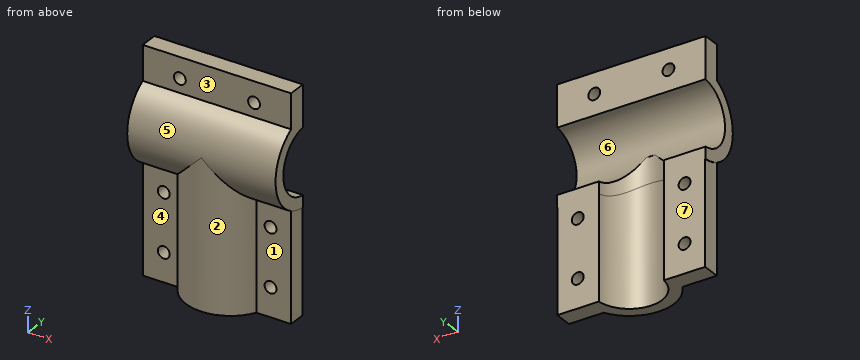
Autodesk Inventor part; units mm, degrees
ref_plane "YZ Plane" through (0, 0, 0) normal (1, 0, 0) x (0, 1, 0)
ref_plane "XZ Plane" through (0, 0, 0) normal (0, 1, 0) x (-1, 0, 0)
ref_plane "XY Plane" through (0, 0, 0) normal (0, 0, 1) x (1, 0, 0)
sketch "Sketch1" plane through (0, 0, 0) normal (1, 0, 0) x (0, 1, 0)
  arc A0 (-1, 14.96663) -> (0, -15) centre (0, 0) ccw
  arc A1 (-1, 10.954451) -> (0, -11) centre (0, 0) ccw
  line L0 (0, 15) -> (0, -15)
  line L1 (-1, 14.96663) -> (-1, 10.954451)
  point P0 (0, 11.5)
  dimension "d0" = 30
  dimension "d1" = 22
extrude "Extrusion1" add sketch "Sketch1" along normal blind 50
sketch "Sketch2" plane through (50, 0, 0) normal (1, 0, 0) x (0, 0, -1)
  line L0 (-10.954451, -1) -> (-14.96663, -1)
  line L1 (-14.96663, -1) -> (-24.96663, -1)
  line L2 (-24.96663, -1) -> (-24.96663, -7)
  line L3 (-24.96663, -7) -> (-13.211534, -7)
  arc A0 (-14.96663, -1) -> (15, 0) centre (0, 0) ccw
  line L4 (-14.96663, -1) -> (-13.211534, -7)
  point P0 (-13.266499, -7)
  dimension "d5" = 10
  dimension "d6" = 6
extrude "Extrusion2" add sketch "Sketch2" against normal blind 50 contours A0 L3 L2 L1
sketch "Sketch3" plane through (0, 0, 0) normal (0, 1, 0) x (-1, 0, 0)
  line L0 (0, 0) -> (-25, 0) construction
  line L1 (-25, 0) -> (-25, -50) construction
  dimension "d9" = 25
  dimension "d10" = 50
ref_plane "Work Plane1" through (25, 0, -50) normal (0, 0, -1) x (-1, 0, 0)
sketch "Sketch4" plane through (25, 0, -50) normal (0, 0, -1) x (-1, 0, 0)
  line L0 (25, 0) -> (-25, 0)
  arc A0 (-10.954451, -1) -> (10.954451, -1) centre (0, 0) ccw
  arc A1 (-14.96663, -1) -> (14.96663, -1) centre (0, 0) ccw
  line L1 (25, -1) -> (-25, -1)
  line L2 (-14.96663, -1) -> (14.96663, -1)
  point P0 (-10.954451, -1)
  point P1 (10.954451, -1)
  dimension "d11" = 22
  dimension "d12" = 30
extrude "Extrusion3" add sketch "Sketch4" against normal up to next contours A0 L1 A1
sketch "Sketch5" plane through (25, 0, -50) normal (0, 0, -1) x (-1, 0, 0)
  arc A0 (-10.954451, -1) -> (10.954451, -1) centre (0, 0) ccw
  circle A1 centre (0, 0) radius 11
  line L0 (25, -1) -> (-25, -1)
  line L1 (14.854796, -1) -> (24.854796, -1)
  arc A2 (-14.96663, -1) -> (0, -15) centre (0, 0) ccw
  line L2 (-14.96663, -1) -> (-24.96663, -1)
  line L3 (-24.96663, -1) -> (-24.96663, -7)
  line L4 (-24.96663, -7) -> (24.854796, -7)
  line L5 (24.854796, -7) -> (24.854796, -1)
  line L6 (-24.96663, -1) -> (24.854796, -1)
  point P0 (25, 0)
  point P1 (-13.266499, -7)
  point P2 (8.485281, -7)
  dimension "d15" = 10
  dimension "d16" = 10
  dimension "d17" = 6
extrude "Extrusion4" add sketch "Sketch5" against normal blind 38.302 contours L0 L5 L4 A0 | A2 L4 L3 L0
sketch "Sketch6" plane through (25, 0, -50) normal (0, 0, -1) x (-1, 0, 0)
  line L0 (25, 0) -> (-25, 0)
  arc A0 (-10.954451, -1) -> (10.954451, -1) centre (0, 0) ccw
  circle A1 centre (0, 0) radius 11
  point P0 (-11, 0)
  point P1 (-10.954451, -1)
  point P2 (11, 0)
extrude "Extrusion5" cut sketch "Sketch6" against normal blind 48.552 contours A1 A0 L0
sketch "Sketch7" plane through (50, 0, -11) normal (0, 1, 0) x (1, 0, 0)
  line L0 (1.146492, -0.964321) -> (-15.803609, -0.964321)
  line L1 (-15.803609, -0.964321) -> (-15.803609, 5.725768)
  line L2 (-15.803609, 5.725768) -> (1.146492, 5.725768)
  line L3 (1.146492, 5.725768) -> (1.146492, -0.964321)
  line L4 (-26.448, -9.552) -> (-36, 0)
  line L5 (-34.667708, -1.332292) -> (-52.233675, -1.332292)
  line L6 (-52.233675, -1.332292) -> (-52.233675, 5.725768)
  line L7 (-52.233675, 5.725768) -> (-34.667708, 5.725768)
  line L8 (-34.667708, 5.725768) -> (-34.667708, -1.332292)
  point P0 (-50, -11)
extrude "Extrusion6" cut sketch "Sketch7" against normal blind 1
sketch "Sketch8" plane through (35.954451, -1, -10.954451) normal (0, 1, 0) x (1, 0, 0)
  line L0 (0, 39.045549) -> (14.012178, 39.045549)
  line L1 (0, 0) -> (-9.506451, -9.506451)
  line L2 (14.012178, 39.045549) -> (14.012178, 4.012178)
  line L3 (0.045549, 19.522774) -> (14.189279, 0.045549) construction
  circle A0 centre (7.117414, 9.784162) radius 2
  line L4 (0.045549, 19.522774) -> (14.012178, 39.045549) construction
  line L5 (0.045549, 19.522774) -> (-21.938424, 19.522774) construction
  line L6 (-21.938424, 19.522774) -> (-35.954451, 39.045549) construction
  line L7 (2.312048, 39.045549) -> (-24.22095, 39.045549) construction
  line L8 (-21.938424, 39.045549) -> (-35.809247, 19.522774) construction
  line L9 (-35.809247, 39.045549) -> (-35.809247, 2.312048) construction
  line L10 (7.117414, 9.784162) -> (-28.873836, 9.784162) construction
  line L11 (-28.873836, 9.784162) -> (-28.873836, 29.284162) construction
  line L12 (-28.873836, 29.284162) -> (7.117414, 29.284162) construction
  line L13 (7.117414, 29.284162) -> (7.117414, 9.784162) construction
  circle A1 centre (-28.873836, 9.784162) radius 2
  circle A2 centre (7.117414, 29.284162) radius 2
  circle A3 centre (-28.873836, 29.284162) radius 2
  line L14 (-35.954451, -21.908902) -> (14.045549, -21.908902) construction
  line L15 (-10.954451, -21.908902) -> (-35.954451, -35.954451) construction
  line L16 (-35.954451, -21.908902) -> (-35.954451, -35.921081)
  line L17 (-10.954451, -35.921081) -> (14.045549, -21.908902) construction
  line L18 (14.045549, -35.921081) -> (-35.954451, -35.921081) construction
  line L19 (14.045549, -35.921081) -> (-10.954451, -21.908902) construction
  circle A4 centre (1.545549, -28.914991) radius 2
  circle A5 centre (-23.454451, -28.914991) radius 2
  point P0 (-35.954451, -10.954451)
  dimension "d24" = 4
  dimension "d25" = 4
  dimension "d26" = 4
  dimension "d27" = 4
  dimension "d28" = 4
  dimension "d29" = 4
extrude "Extrusion7" cut sketch "Sketch8" against normal blind 48.552
properties part number "betterTconection"
Check sheet for the modelled part. Datum: model origin and axes. Units: mm. Face numbers are marked on the shaded views. A direction names the side the tool comes from. Give positions to 0.01 mm unless a question says otherwise; leave off trailing zeros. Loops run counter-clockwise (first coordinate to the right, second up) from the corner with the lowest first, then second, coordinate; pieces in that order, holes last. Notation, with made-up numbers: M -27,36 L -10,36 A12 ccw -10,55 Z; hole C 27.5,80.25 d7. An arc over 180 degrees is marked long. Return JSON: item names as keys, results as strings. Group by question number.
1. Mould release check, pull along Z, two halves, no side actions. Record for the marked faces 5, 6 and 7: released by +Z, released by -Z, zero draft, split by the parting line, or undercut.
2. Cross-section at B-B on x = 37.5. Record the boundary of the cut face in (y, z), plus the area to 3 significant figures.
3. Cross-section at A-A on y = -4.5. State how many separate pieces and enclosed holes the cut face has, plus the area to 3 significant figures.
4. Thickness scan on L1, parallel to X at y = -6.25, z = -19.5; L2, parallel to Z at x = 36.5, y = -5.75; L3, parallel to X at y = -2.75, z = -41. Record the ranges inside material, lowest first.
5. Go/stop test with flat-tipped pins: pin 1 (9.5 mm diameter, centred on x = 46.5, z = -25, fed in from -Y); pin 2 (2 mm diameter, centred on x = 28, z = -16, fed in from +Y); pin 3 (2 mm diameter, centred on x = 32, y = -12, fed in from +Z); pin 4 (3 mm diameter, centred on x = 37.5, z = 17.96, fed in from -Y). Record where each tip stops, or that it passes through.
6. Cross-section at D-D on y = -12.5. Record the boundary of the cut face in (x, z).
7. Cross-section at C-C on y = -8.75. Record the boundary of the cut face in (x, z), plus the area to 3 significant figures.
8. Tool access check on the marked faces 1, 2, 3 and 4. Record the directions out of +Z, -Z, +X, -X, +Y, -Y that give a thin tool (end or side, any length) a straight path to the whole face; none if there is none.
Return value:
{
 "1": {"face 5": "split by the parting line", "face 6": "undercut", "face 7": "zero draft"},
 "2": {"outline": "M -8.29,-50 L -1,-50 L -1,-10.95 A11 cw -1,10.95 L -1,15.96 L -7,15.96 L -7,13.27 A15 ccw -8.29,-12.5 Z; M -7,19.96 L -1,19.96 L -1,24.97 L -7,24.97 Z", "area": "457 mm^2"},
 "3": {"separate pieces": "3", "enclosed holes": "6", "area": "1,860 mm^2"},
 "4": {"L1": "0.15 to 5.51, 8.65 to 15.95, 34.05 to 41.5, 44.64 to 49.97", "L2": "-50 to -9.38, 9.38 to 16.23, 19.69 to 24.97", "L3": "0.15 to 5.23, 8.93 to 14.35, 35.65 to 41.22, 44.92 to 49.97"},
 "5": {"pin 1": "y = -7", "pin 2": "y = -10.25", "pin 3": "z = 10.2", "pin 4": "through"},
 "6": {"outline": "M 0,-8.29 L 16.71,-8.29 L 16.71,-50 L 33.29,-50 L 33.29,-8.29 L 50,-8.29 L 50,8.29 L 0,8.29 Z"},
 "7": {"outline": "M 0,-12.18 L 12.82,-12.18 L 12.82,-50 L 18.33,-50 L 18.33,-6.67 L 0,-6.67 Z; M 0,6.67 L 50,6.67 L 50,12.18 L 0,12.18 Z; M 31.67,-50 L 37.18,-50 L 37.18,-12.18 L 50,-12.18 L 50,-6.67 L 31.67,-6.67 Z", "area": "895 mm^2"},
 "8": {"face 1": "-Z, +X, -Y", "face 2": "-Z, -Y", "face 3": "+Z, +X, -X, -Y", "face 4": "-Z, -X, -Y"}
}
